Autodesk Inventor part; units mm, degrees
ref_plane "YZ Plane" through (0, 0, 0) normal (1, 0, 0) x (0, 1, 0)
ref_plane "XZ Plane" through (0, 0, 0) normal (0, 1, 0) x (-1, 0, 0)
ref_plane "XY Plane" through (0, 0, 0) normal (0, 0, 1) x (1, 0, 0)
sketch "Sketch1" plane through (0, 0, 0) normal (0, 0, 1) x (1, 0, 0)
  line L0 (60, -75) -> (-60, -75)
  line L1 (-60, -75) -> (-60, 75)
  line L2 (-60, 75) -> (60, 75)
  line L3 (60, 75) -> (60, -75)
  line L4 (60, 75) -> (-60, -75) construction
  point P0 (0, 0)
  point P1 (0, 0)
  dimension "d1" = 150
  dimension "d2" = 120
extrude "Plate1" add sketch "Sketch1" along normal blind 3
sketch "Sketch2" plane through (0, 0, 0) normal (0, 0, 1) x (1, 0, 0)
  circle A0 centre (0, 0) radius 17.5
  line L0 (35, -32.5) -> (-35, -32.5) construction
  line L1 (-35, -32.5) -> (-35, 32.5) construction
  line L2 (-35, 32.5) -> (35, 32.5) construction
  line L3 (35, 32.5) -> (35, -32.5) construction
  line L4 (35, -32.5) -> (-35, 32.5) construction
  line L5 (-35, -32.5) -> (35, 32.5) construction
  circle A1 centre (-35, -32.5) radius 4
  circle A2 centre (35, -32.5) radius 4
  circle A3 centre (35, 32.5) radius 4
  circle A4 centre (-35, 32.5) radius 4
  circle A5 centre (0, 50) radius 4
  circle A6 centre (0, -50) radius 4
  line L6 (35, 0) -> (-35, 0) construction
  point P0 (75, 0)
  point P1 (0, 0)
  dimension "d3" = 35
  dimension "d4" = 70
  dimension "d5" = 65
  dimension "d7" = 8
  dimension "d32" = 100
extrude "Extrusion1" cut sketch "Sketch2" along normal through all contours A1 | A2 | A3 | A4 | A5 | A6
sketch "Sketch3" plane through (-57, 75, 3) normal (-1, 0, 0) x (0, -1, 0)
  line L0 (150, 0) -> (0, 0)
  line L1 (0, 0) -> (0, -20)
  line L2 (0, -20) -> (150, -20)
  line L3 (150, -20) -> (150, 0)
edge flange "Flange1" height 20 angle 90 thickness 3 bend radius 3 thickness toward (-1, 0, 0) relief tear relief width 3 relief depth 1.5 corner gap 3 corner form 0 edges at (-60, 0, 0) (60, 0, 0) wall of the first edge with corners at (-57, -75, 3) (-57, 75, 3) (-57, 75, -17) (-57, -75, -17)
bend "Bend1"
corner "Corner1"
sketch "Sketch4" plane through (0, 0, 0) normal (0, 0, 1) x (1, 0, 0)
  circle A0 centre (0, 75) radius 17.5
  line L0 (0, 125) -> (0, 105) construction
  line L1 (-3, 125) -> (-3, 105)
  line L2 (3, 105) -> (3, 125)
  arc A1 (3, 125) -> (-3, 125) centre (0, 125) ccw
  arc A2 (-3, 105) -> (3, 105) centre (0, 105) ccw
  arc A3 (34.641, 95) -> (20, 109.641) centre (0, 75) ccw construction
  arc A4 (37.2391, 96.5) -> (21.5, 112.2391) centre (0, 75) ccw
  arc A5 (32.0429, 93.5) -> (18.5, 107.0429) centre (0, 75) ccw
  arc A6 (32.0429, 93.5) -> (37.2391, 96.5) centre (34.641, 95) ccw
  arc A7 (21.5, 112.2391) -> (18.5, 107.0429) centre (20, 109.641) ccw
  line L3 (0, 75) -> (20, 109.641) construction
  line L4 (0, 75) -> (40, 75) construction
  line L5 (0, 75) -> (34.641, 95) construction
  point P0 (0, 0)
  point P1 (0, 115)
  dimension "d20" = 20
  dimension "d21" = 6
  dimension "d22" = 30
  dimension "d23" = 60
  dimension "d24" = 30
  dimension "d25" = 6
  dimension "d26" = 40
extrude "Extrusion2" [suppressed]
pattern_circular "Circular Pattern1" [suppressed]
equation "\"d0\" = Thickness"
equation "\"d10\" = BendReliefWidth"
equation "\"d11\" = BendReliefDepth"
equation "\"d12\" = MinimumRemnant"
equation "\"d13\" = TransitionRadius"
equation "\"d16\" = BendRadius"
equation "\"d17\" = CornerReliefSize"
equation "\"d18\" = GapSize"
equation "\"d19\" = JacobiRadiusSize"
equation "\"BendRadius\" = Thickness"
equation "\"BendReliefWidth\" = Thickness"
equation "\"BendReliefDepth\" = 0.5 * Thickness"
equation "\"CornerReliefSize\" = 4 * Thickness"
equation "\"MinimumRemnant\" = 2 * Thickness"
equation "\"TransitionRadius\" = BendRadius"
equation "\"JacobiRadiusSize\" = BendRadius"
equation "\"GapSize\" = Thickness"
properties part number "FL3.6.2  Motor pillar" material "Stainless Steel"
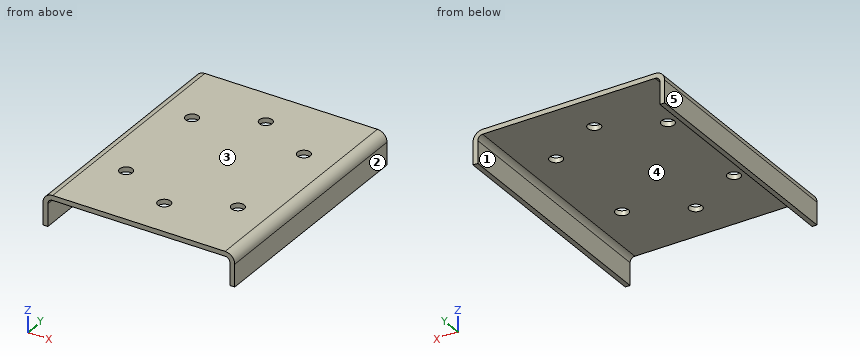
Read the model definition and answer for the solid it produces. Units are mm, in the model's axes. Face numbers are marked on the shaded views. A direction names the side the tool comes from. Give positions to 0.01 mm unless a question says otherwise; leave off trailing zeros. Loops run counter-clockwise (first coordinate to the right, second up) from the corner with the lowest first, then second, coordinate; pieces in that order, holes last.
Item 1: This flat-tipped pin is pushed along its axis until it touches: pin 1 Ø10.5 at (x, y) = (-35, -32.5) entering from -Z. Where does it stop, or does it pass through?
Item 2: The part is cut by section A-A (y = 32.5). Write down the section's boundary in (x, z), and give its area (3 significant figures).
Item 3: The part is cut by section C-C (y = -50). Write down the section's boundary in (x, z).
Item 4: For the marked faces 4 and 5, determine the directions among +Z, -Z, +X, -X, +Y, -Y from which every point of the face is accessible in a straight line to the end or side of a thin tool.
Item 5: The part is cut by section B-B (x = 35). Write down the section's boundary in (y, z), and give its area (3 significant figures).
Item 6: The part is cut by section D-D (z = -7). Write down the section's boundary in (x, y).
Item 7: The mould has two halves that part along X. Classify the marked faces 1, 2 and 3: released by +X, released by -X, zero draft, split by the parting line, or undercut.
Item 8: Find the intervals of material crossed by line 1 along Y through (x, z) = (-35, 1.5); line 2 along Y through (x, z) = (0, 2.15); line 3 along X through (y, z) = (30.5, -9.5), in increasing order.
Taken from the geometry:
1. pin 1: stops at z = 0
2. outline: (-60, -17) - (-57, -17) - (-57, -3) arc R3 cw to (-54, 0) - (-39, 0) - (-39, 3) - (-54, 3) arc R6 ccw to (-60, -3) - close; (-31, 0) - (31, 0) - (31, 3) - (-31, 3) - close; (39, 0) - (54, 0) arc R3 cw to (57, -3) - (57, -17) - (60, -17) - (60, -3) arc R6 ccw to (54, 3) - (39, 3) - close
2. area: 402 mm2
3. outline: (-60, -17) - (-57, -17) - (-57, -3) arc R3 cw to (-54, 0) - (-4, 0) - (-4, 3) - (-54, 3) arc R6 ccw to (-60, -3) - close; (4, 0) - (54, 0) arc R3 cw to (57, -3) - (57, -17) - (60, -17) - (60, -3) arc R6 ccw to (54, 3) - (4, 3) - close
4. face 4: -Z, +Y, -Y
4. face 5: +Z, -Z, -X, +Y, -Y
5. outline: (-75, 0) - (-36.5, 0) - (-36.5, 3) - (-75, 3) - close; (-28.5, 0) - (28.5, 0) - (28.5, 3) - (-28.5, 3) - close; (36.5, 0) - (75, 0) - (75, 3) - (36.5, 3) - close
5. area: 402 mm2
6. outline: (-60, -75) - (-57, -75) - (-57, 75) - (-60, 75) - close; (57, -75) - (60, -75) - (60, 75) - (57, 75) - close
7. face 1: undercut
7. face 2: released by +X
7. face 3: zero draft
8. line 1: y = -75 to -36.5, -28.5 to 28.5, 36.5 to 75
8. line 2: y = -75 to -54, -46 to 46, 54 to 75
8. line 3: x = -60 to -57, 57 to 60
